Here's how the part is built. I have some questions about the finished solid (model axes, mm). A direction names the side the tool comes from. Round coordinates to 2 decimals unless told otherwise and drop trailing zeros. Write each loop counter-clockwise with the first axis right and the second up, starting at its lowest first coordinate (ties: lowest second). Pieces come first, ordered by that corner, then holes. Notation, with made-up numbers: (-2, 87) -> (56, 87) arc R20 cw to (56, 113) -> close; hole circle Ø1 at (-38, 23). An arc over 180 degrees is marked (long way). Answer as CSV lines item,"result".
from build123d import *

# Parameters (mm, degrees)
F0_R      = 19.1564129226
F1_DEPTH  = 25.4
F2_W      = 127.5142282248
F2_H      = 41.1144047976
F3_DEPTH  = 50.8
F5_DEPTH  = 59.6617998013
F7_DEPTH  = 21.8189658163
F8_R      = 11.5269990365
F9_DEPTH  = 234.9744529853
F11_DEPTH = 21.8189658163


with BuildPart() as f1:
    # F0 (on Top) → F1 (new body)
    with BuildSketch(Plane.XY):
        with BuildLine():
            ThreePointArc((132.1127414703, -39.1035974026), (171.2163388729, 0), (132.1127414703, 39.1035974026))
            Line((132.1127414703, 39.1035974026), (-132.1127414703, 39.1035974026))
            ThreePointArc((-132.1127414703, 39.1035974026), (-171.2163388729, 0), (-132.1127414703, -39.1035974026))
            Line((-132.1127414703, -39.1035974026), (132.1127414703, -39.1035974026))
        make_face()
        with Locations((-132.1127414703, 0)):
            Circle(F0_R, mode=Mode.SUBTRACT)
        with Locations((132.1127414703, 0)):
            Circle(F0_R, mode=Mode.SUBTRACT)
    extrude(amount=F1_DEPTH)

    # F2 (on face) → F3 (join)
    with BuildSketch(Plane.XY.offset(25.4)):
        Rectangle(F2_W, F2_H)
    extrude(amount=F3_DEPTH)

    # F4 (on face) → F5 (cut, through all)
    with BuildSketch(Plane.XZ.offset(20.5572023988)):
        with BuildLine():
            ThreePointArc((-41.9381482961, 76.2), (0, 34.2618517039), (41.9381482961, 76.2))
            Line((41.9381482961, 76.2), (-41.9381482961, 76.2))
        make_face()
    extrude(amount=-F5_DEPTH, mode=Mode.SUBTRACT)

    # F6 (on face) → F7 (join, through all)
    with BuildSketch(Plane(origin=(-63.7571141124, 0, 0), x_dir=(0, -1, 0), z_dir=(-1, 0, 0))):
        with BuildLine():
            Line((-20.5572023988, 76.2), (20.5572023988, 76.2))
            ThreePointArc((20.5572023988, 76.2), (0, 96.7572023988), (-20.5572023988, 76.2))
        make_face()
    extrude(amount=-F7_DEPTH)

    # F8 (on face) → F9 (cut, through all)
    with BuildSketch(Plane(origin=(-63.7571141124, 0, 0), x_dir=(0, -1, 0), z_dir=(-1, 0, 0))):
        with Locations((0, 76.2)):
            Circle(F8_R)
    extrude(amount=-F9_DEPTH, mode=Mode.SUBTRACT)

    # F10 (on face) → F11 (join, through all)
    with BuildSketch(Plane.YZ.offset(63.7571141124)):
        with BuildLine():
            ThreePointArc((20.5572023988, 76.2), (0, 96.7572023988), (-20.5572023988, 76.2))
            Line((-20.5572023988, 76.2), (-11.5269990365, 76.2))
            ThreePointArc((-11.5269990365, 76.2), (0, 87.7269990365), (11.5269990365, 76.2))
            Line((11.5269990365, 76.2), (20.5572023988, 76.2))
        make_face()
    extrude(amount=-F11_DEPTH)


solid = f1.part
Item 1: I need wall thicknesses on L1, parallel to Z at x = -51.25, y = 0; L2, parallel to X at y = -16, z = 11; L3, parallel to X at y = 2, z = 20. Which ranges of each line are inside material? Lowest first, please.
Results found:
L1,"z = 0 to 64.67, 87.73 to 96.76"
L2,"x = -167.79 to -142.65, -121.58 to 121.58, 142.65 to 167.79"
L3,"x = -171.17 to -151.16, -113.06 to 113.06, 151.16 to 171.17"
Item 2: Suppose I cut it at D-D, the plane z = 13.5. List the corners of the cut face in (x, y) for me, then the cut area to 3 significant figures.
Results found:
outline,"(-132.11, -39.1) -> (132.11, -39.1) arc R39.1 ccw to (132.11, 39.1) -> (-132.11, 39.1) arc R39.1 ccw to start; hole circle Ø38.31 at (-132.11, 0); hole circle Ø38.31 at (132.11, 0)"
area,"23,200 mm²"
Item 3: Suppose I cut it at B-B, the plane z = 50. List the corners of the cut face in (x, y) for me, then the cut area to 3 significant figures.
Results found:
outline,"(-63.76, -20.56) -> (-32.75, -20.56) -> (-32.75, 20.56) -> (-63.76, 20.56) -> close; (32.75, -20.56) -> (63.76, -20.56) -> (63.76, 20.56) -> (32.75, 20.56) -> close"
area,"2,550 mm²"
Item 4: For faces 1 (the flat face through (-1, 20.557, 34)), 2 (the flat face through (-1, -20.557, 34)), 3 (the cylindrical face through (52.204, 2.499, 64.947)), 4 (the flat face through (63.757, 0, 54)), 5 (the flat face through (-63.757, 0, 54)), which set-ups out of +Z, -Z, +X, -X, +Y, -Y let a thin tool reach every point of the face, with its end or its side?
Results found:
face 1,"+Z, +X, -X, +Y"
face 2,"+Z, +X, -X, -Y"
face 3,"+X, -X"
face 4,"+Z, +X, +Y, -Y"
face 5,"+Z, -X, +Y, -Y"
Item 5: Will these pins go through, and if not, where does the flat tip stop? pin 1 (5 mm diameter, centred on x = -136.5, y = 18.5, fed in from -Z); pin 2 (14 mm diameter, centred on y = 0, z = 76.2, fed in from +X); pin 3 (2 mm diameter, centred on x = 18.5, y = -22, fed in from +Z); pin 4 (10 mm diameter, centred on y = -21.5, z = 72.5, fed in from +X).
Results found:
pin 1,"stops at z = 0"
pin 2,"passes through"
pin 3,"stops at z = 25.4"
pin 4,"stops at x = 63.76"
Item 6: Suppose I cut it at C-C, the plane x = -140. List the corners of the cut face in (y, z) for me.
Results found:
outline,"(-38.3, 0) -> (-17.46, 0) -> (-17.46, 25.4) -> (-38.3, 25.4) -> close; (17.46, 0) -> (38.3, 0) -> (38.3, 25.4) -> (17.46, 25.4) -> close"
Item 7: If we mould it in two halves opening along X, with no side actions, what happens to faces 6 (the flat face through (-41.938, 0, 89)), 7 (the cylindrical face through (-171.207, 0.86, 12.522)), 8 (the flat face through (-2, 1, 0)), 9 (the flat face through (41.938, 0, 89))? For each: pulls with the +X half, pulls with the -X half, needs draft (parallel to the pull), parting line crosses it, or undercut.
Results found:
face 6,"undercut"
face 7,"pulls with the -X half"
face 8,"needs draft"
face 9,"undercut"
Item 8: Suppose I cut it at A-A, the plane y = 0. List the corners of the cut face in (x, z) for me, then the cut area to 3 significant figures.
Results found:
outline,"(-171.22, 0) -> (-151.27, 0) -> (-151.27, 25.4) -> (-171.22, 25.4) -> close; (-112.96, 0) -> (112.96, 0) -> (112.96, 25.4) -> (63.76, 25.4) -> (63.76, 64.67) -> (40.32, 64.67) arc R41.94 cw to (-40.32, 64.67) -> (-63.76, 64.67) -> (-63.76, 25.4) -> (-112.96, 25.4) -> close; (-63.76, 87.73) -> (-41.94, 87.73) -> (-41.94, 96.76) -> (-63.76, 96.76) -> close; (41.94, 87.73) -> (63.76, 87.73) -> (63.76, 96.76) -> (41.94, 96.76) -> close; (151.27, 0) -> (171.22, 0) -> (171.22, 25.4) -> (151.27, 25.4) -> close"
area,"10,300 mm²"
